```python
from build123d import *

# Parameters (mm, degrees)
BOSS_EXTRUDE1_DEPTH = 75
SKETCH2_R           = 2
CUT_EXTRUDE1_DEPTH  = 10
CUT_EXTRUDE2_DEPTH  = 10
CHAMFER1_SIZE       = 2
SKETCH3_R           = 2.543008444
BOSS_EXTRUDE2_DEPTH = 40


with BuildPart() as part:
    # Sketch1 → Boss-Extrude1 (new body)
    with BuildSketch(Plane(origin=(0, 0, 0), x_dir=(0, 0, -1), z_dir=(1, 0, 0))):
        Polygon((-35.447605249, 4.173188871), (35.206481481, 4.173188871), (35.206481481, 14.173188871), (14.511910864, 14.173188871), (8.571096195, 24.699446456), align=None)
    extrude(amount=BOSS_EXTRUDE1_DEPTH)

    # Sketch2 → Cut-Extrude1 (cut)
    with BuildSketch(Plane(origin=(0, 14.173188871, 0), x_dir=(1, 0, 0), z_dir=(0, 1, 0))):
        with Locations(Location((5, 25.374559272, 0), (0, 0, 270))):
            Circle(SKETCH2_R)
        with Locations(Location((69.999998955, 25.38621548, 0), (0, 0, 270))):
            Circle(SKETCH2_R)
    extrude(amount=-CUT_EXTRUDE1_DEPTH, mode=Mode.SUBTRACT)

    # Sketch4 → Cut-Extrude2 (cut)
    with BuildSketch(Plane(origin=(0, 17.005051997, 7.929585973), x_dir=(1, 0, 0), z_dir=(0, 0.9063077870366527, 0.4226182617406937))):
        Polygon((0, -30.362774842), (7.065850082, -25.103103439), (13.976560291, -30.362774842), align=None)
        Polygon((22.065850082, -25.103103439), (28.976560291, -30.362774842), (15, -30.362774842), align=None)
        Polygon((37.065850082, -25.103103439), (43.976560291, -30.362774842), (30, -30.362774842), align=None)
        Polygon((52.065850082, -25.103103439), (58.976560291, -30.362774842), (45, -30.362774842), align=None)
        Polygon((67.065850082, -25.103103439), (73.976560291, -30.362774842), (60, -30.362774842), align=None)
    extrude(amount=-CUT_EXTRUDE2_DEPTH, mode=Mode.SUBTRACT)

    # Chamfer1
    chamfer1_edges = [part.edges().sort_by_distance(p)[0] for p in [
        (5, 4.173188871, -27.374559272),
        (69.999998955, 4.173188871, -27.38621548),
    ]]
    chamfer(chamfer1_edges, length=CHAMFER1_SIZE)

    # Sketch3 → Boss-Extrude2 (add)
    with BuildSketch(Plane.ZY):
        with Locations((-5.547587106, 8.033515635)):
            Circle(SKETCH3_R)
    extrude(amount=BOSS_EXTRUDE2_DEPTH)


solid = part.part
```
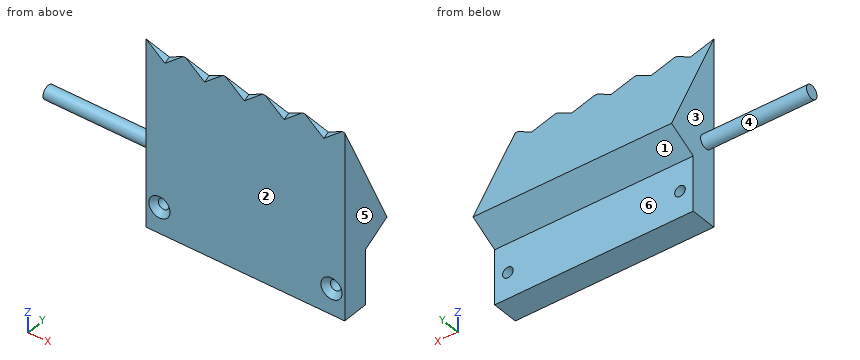
Can you work these out from the model? Positions are in its coordinate system, mm. Face numbers are marked on the shaded views. A direction names the side the tool comes from. Round coordinates to 2 decimals unless told otherwise and drop trailing zeros. Loops run counter-clockwise (first coordinate to the right, second up) from the corner with the lowest first, then second, coordinate; pieces in that order, holes last.
Item 1: Will these pins go through, and if not, where does the flat tip stop? pin 1 Ø10 at (y, z) = (19, 6.5) entering from -X; pin 2 Ø23 at (x, z) = (51.5, -27.5) entering from +Y; pin 3 Ø6.5 at (x, z) = (5, -25.37) entering from -Y.
Item 2: Suppose I cut it at D-D, the plane z = 23. Write out the boundary of the cut face in (x, y), then the cut area to 3 significant figures.
Item 3: Which directions (+Z, -Z, +X, -X, +Y, -Y) give clear straight access to the entire face, cutting with the end or side of a thin tool? Please do the marked faces 5 and 6.
Item 4: Suppose I cut it at A-A, the plane x = 5. Write out the boundary of the cut face in (y, z).
Item 5: Suppose I cut it at C-C, the plane x = 32. Write out the boundary of the cut face in (y, z).
Item 6: Suppose I cut it at B-B, the plane y = 12. Write out the boundary of the cut face in (x, z).
Item 7: Please list where these lines run through material, in increasing order: L1, parallel to Y at x = 26, z = -27; L2, parallel to X at y = 15.75, z = -10.5; L3, parallel to Z at x = 36, y = 23.5.
Item 8: If we mould it in two halves opening along Y, with no side actions, what happens to the marked faces 1, 2, 3 and 4? For each: +Y half, -Y half, draft (parallel to the pull), parting line (faces both ways), or undercut.
Reported:
1. pin 1: stops at x = 0
1. pin 2: stops at y = 14.17
1. pin 3: stops at y = 4.92
2. outline: (0, 4.17) - (75, 4.17) - (75, 9.98) - (0, 9.98) - close
2. area: 435 mm2
3. face 5: +Z, -Z, +X, +Y, -Y
3. face 6: -Z, +X, -X, +Y
4. outline: (4.17, -35.21) - (14.17, -35.21) - (14.17, -27.37) - (6.17, -27.37) - (4.17, -29.37) - close; (4.17, -21.37) - (6.17, -23.37) - (14.17, -23.37) - (14.17, -14.51) - (24.7, -8.57) - (5.75, 32.07) - (4.17, 31.34) - close
5. outline: (4.17, -35.21) - (14.17, -35.21) - (14.17, -14.51) - (24.7, -8.57) - (4.8, 34.1) - (4.17, 33.8) - close
6. outline: (0, -35.21) - (75, -35.21) - (75, 18.66) - (0, 18.66) - close; hole circle Ø4 at (5, -25.37); hole circle Ø4 at (70, -25.39)
7. L1: y = 4.17 to 14.17
7. L2: x = 0 to 75
7. L3: z = -9.25 to -6
8. face 1: +Y half
8. face 2: -Y half
8. face 3: draft
8. face 4: parting line
